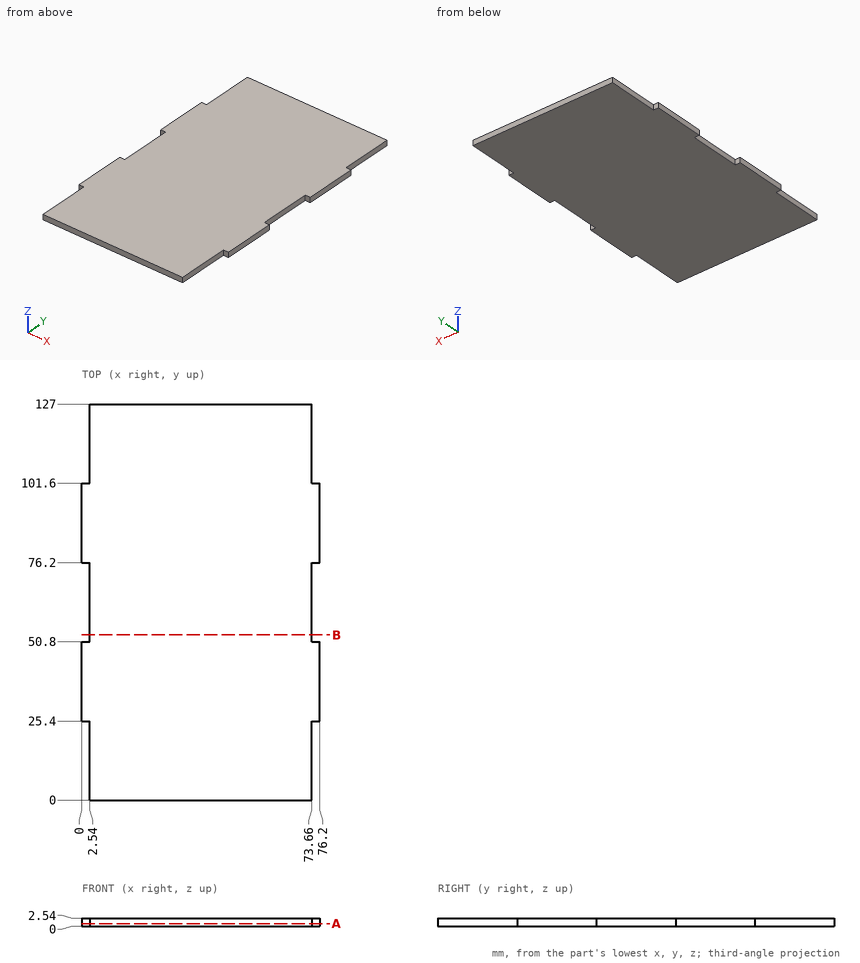
Source: three-view drawing plus pictorial views. Frame: mm from the lowest corner of the part. Give positions to 0.01 mm unless a question says otherwise; leave off trailing zeros. Loops run counter-clockwise (first coordinate to the right, second up) from the corner with the lowest first, then second, coordinate; pieces in that order, holes last.
1) Section query A-A on z = 0.8. Return the cut outline in (x, y).
A:
outline: (0, 25.4) - (2.54, 25.4) - (2.54, 0) - (73.66, 0) - (73.66, 25.4) - (76.2, 25.4) - (76.2, 50.8) - (73.66, 50.8) - (73.66, 76.2) - (76.2, 76.2) - (76.2, 101.6) - (73.66, 101.6) - (73.66, 127) - (2.54, 127) - (2.54, 101.6) - (0, 101.6) - (0, 76.2) - (2.54, 76.2) - (2.54, 50.8) - (0, 50.8) - close
2) Contact query for flat-ended pins moving along their axis: pin 1 (0.8 mm diameter, centred on x = 1.5, z = 1, fed in from -Y); pin 2 (0.8 mm diameter, centred on y = 114.5, z = 0.5, fed in from -X); pin 3 (1.3 mm diameter, centred on x = 1.5, z = 1.5, fed in from +Y). Output: stop coordinate, or through.
A:
pin 1: stops at y = 25.4
pin 2: stops at x = 2.54
pin 3: stops at y = 101.6
3) Section query B-B on y = 53. Return the cut outline in (x, z).
A:
outline: (2.54, 0) - (73.66, 0) - (73.66, 2.54) - (2.54, 2.54) - close
4) Line query: L1, parallel to X at y = 12, z = 1.4. Output: solid intervals per line, ascending.
A:
L1: x = 2.54 to 73.66
